Can you work these out from the model? Positions are in its coordinate system, mm. Face numbers are marked on the shaded views. A direction names the side the tool comes from. Give positions to 0.01 mm unless a question says otherwise; leave off trailing zeros. Loops run counter-clockwise (first coordinate to the right, second up) from the corner with the lowest first, then second, coordinate; pieces in that order, holes last. Notation, with made-up numbers: (86, 76.5) - (96, 76.5) arc R31 ccw to (96, 115.5) - close; hole circle Ø1 at (-18.75, -21.5). An arc over 180 degrees is marked (long way). Answer as a JSON object with one key per item and string values.
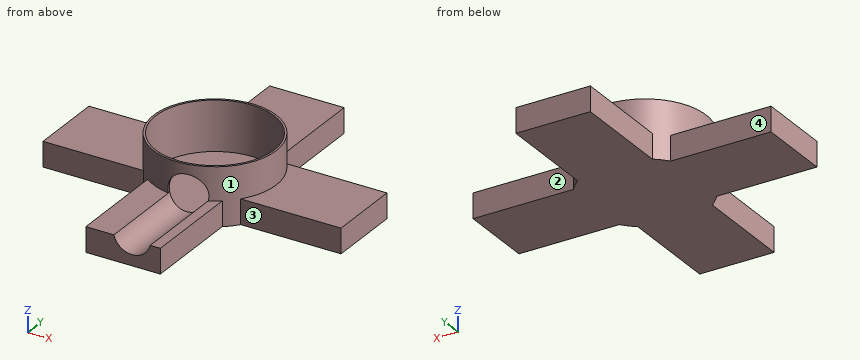
Autodesk Inventor part; units mm, degrees
ref_plane "YZ Plane" through (0, 0, 0) normal (1, 0, 0) x (0, 1, 0)
ref_plane "XZ Plane" through (0, 0, 0) normal (0, 1, 0) x (-1, 0, 0)
ref_plane "XY Plane" through (0, 0, 0) normal (0, 0, 1) x (1, 0, 0)
sketch "Sketch1" plane through (0, 0, 0) normal (0, 0, 1) x (1, 0, 0)
  circle A0 centre (0, 0) radius 35.75
  circle A1 centre (0, 0) radius 37
  line L0 (-22.5, -90) -> (-22.5, 90)
  line L1 (-22.5, 90) -> (22.5, 90)
  line L2 (22.5, 90) -> (22.5, -90)
  line L3 (22.5, -90) -> (-22.5, -90)
  line L4 (-22.5, -90) -> (22.5, 90) construction
  line L5 (-22.5, 90) -> (22.5, -90) construction
  line L6 (-90, 22.5) -> (90, 22.5)
  line L7 (90, 22.5) -> (90, -22.5)
  line L8 (90, -22.5) -> (-90, -22.5)
  line L9 (-90, -22.5) -> (-90, 22.5)
  line L10 (-90, 22.5) -> (90, -22.5) construction
  line L11 (90, 22.5) -> (-90, -22.5) construction
  point P0 (22.5, -29.3726)
  point P1 (-22.5, -29.3726)
  point P2 (-29.3726, -22.5)
  point P3 (-29.3726, 22.5)
  point P4 (-22.5, 29.3726)
  point P5 (22.5, 29.3726)
  point P6 (29.3726, 22.5)
  point P7 (29.3726, -22.5)
  dimension "d0" = 71.5
  dimension "d1" = 74
  dimension "d2" = 180
  dimension "d3" = 45
  dimension "d4" = 180
  dimension "d5" = 45
extrude "Extrusion1" add sketch "Sketch1" along normal blind 5 contours A0 L8 L2 L6 | L6 L2 A0 | A0 L2 L8 | L2 L6 L0 A0 | L2 L8 L0 L6 | A0 L0 L8 L2 | L0 L6 A0 | L0 L8 A0 L6 | A0 L8 L0
extrude "Extrusion2" add sketch "Sketch1" along normal blind 30 contours A0 L6 A1 L8 | A0 L2 A1 L6 | L8 A1 L2 A0 | A0 L0 A1 L2 | L2 A1 L0 A0 | A0 L6 A1 L0 | L0 A1 L8 A0 | A0 L8 A1 L6
extrude "Extrusion3" add sketch "Sketch1" along normal blind 15 contours L6 L7 L8 A1 | A1 L0 L1 L2 | L2 L3 L0 A1 | A1 L8 L9 L6
sketch "Sketch2" plane through (-22.5, -90, 0) normal (0, -1, 0) x (1, 0, 0)
  point P0 (22.5, 0)
  point P1 (27.9129, 17.8091)
hole "Hole1" at (5.4129, -90, 17.8091) direction (0, 1, 0) diameter 22.606 depth 88.75 tip angle 118
move faces "Move1" translate (0, 0, 5) faces at (-36.0055, 0, 30)
equation "\"BendRadius\" = Thickness"
equation "\"BendReliefWidth\" = Thickness"
equation "\"BendReliefDepth\" = 0.5 * Thickness"
equation "\"CornerReliefSize\" = 4 * Thickness"
equation "\"MinimumRemnant\" = 2 * Thickness"
equation "\"TransitionRadius\" = BendRadius"
equation "\"JacobiRadiusSize\" = BendRadius"
equation "\"GapSize\" = Thickness"
1) Which directions (+Z, -Z, +X, -X, +Y, -Y) give clear straight access to the entire face, cutting with the end or side of a thin tool? Please do the marked faces 1, 2, 3 and 4.
Check sheet entries:
{"face 1": "+Z", "face 2": "+Z, -Z, +X, +Y", "face 3": "+Z, -Z, +X, -Y", "face 4": "+Z, -Z, -X, +Y"}
2) I need wall thicknesses on L1, parallel to X at y = 0, z = 12; L2, parallel to Y at x = 0, z = 28; L3, parallel to Z at x = 6, y = 22.5. Which ranges of each line are inside material? Lowest first, please.
Check sheet entries:
{"L1": "-90 to -35.75, 35.75 to 90", "L2": "-37 to -35.75, 35.75 to 37", "L3": "0 to 5"}
3) I'm going to push flat-ended pins straight in: P1, Ø12, axis at y = -62, z = 4, coming from the +X side; P2, Ø20.5, axis at x = 5.41, z = 17.81, coming from the -Y side; P3, Ø7.5, axis at y = -71, z = 6, coming from the -X side. Where does each tip first touch, or does it pass through?
Check sheet entries:
{"P1": "x = 22.5", "P2": "y = 32.14", "P3": "x = -22.5"}
4) Imagine slicing it at C-C on z = 32. Write out the boundary of the cut face in (x, y), and give its area (3 significant figures).
Check sheet entries:
{"outline": "circle Ø74 at (0, 0); hole circle Ø71.5 at (0, 0)", "area": "286 mm2"}
5) Imagine slicing it at D-D on z = 10. Write out the boundary of the cut face in (x, y), and give its area (3 significant figures).
Check sheet entries:
{"outline": "(-90, -22.5) - (-29.37, -22.5) arc R37 ccw to (-22.5, -29.37) - (-22.5, -90) - (-2.76, -90) - (-2.76, -35.64) arc R35.75 cw (long way) to (13.58, -33.07) - (13.58, -90) - (22.5, -90) - (22.5, -29.37) arc R37 ccw to (29.37, -22.5) - (90, -22.5) - (90, 22.5) - (29.37, 22.5) arc R37 ccw to (22.5, 29.37) - (22.5, 90) - (-22.5, 90) - (-22.5, 29.37) arc R37 ccw to (-29.37, 22.5) - (-90, 22.5) - close", "area": "9,360 mm2"}
6) Imagine slicing it at B-B on y = 0. Write out the boundary of the cut face in (x, z).
Check sheet entries:
{"outline": "(-90, 0) - (90, 0) - (90, 15) - (37, 15) - (37, 35) - (35.75, 35) - (35.75, 5) - (-35.75, 5) - (-35.75, 35) - (-37, 35) - (-37, 15) - (-90, 15) - close"}
7) Imagine slicing it at A-A on x = 0. Write out the boundary of the cut face in (y, z), and give its area (3 significant figures).
Check sheet entries:
{"outline": "(-90, 0) - (90, 0) - (90, 15) - (37, 15) - (37, 35) - (35.75, 35) - (35.75, 5) - (-35.75, 5) - (-35.75, 7.89) - (-90, 7.89) - close; (-37, 27.73) - (-35.75, 27.73) - (-35.75, 35) - (-37, 35) - close", "area": "1,630 mm2"}
